from build123d import *

# Parameters (mm, degrees)
SKETCH1_R           = 12.5
BOSS_EXTRUDE1_DEPTH = 3
SKETCH3_R           = 5
BOSS_EXTRUDE2_DEPTH = 3
CUT_EXTRUDE1_DEPTH  = 10


with BuildPart() as part:
    # Sketch1 → Boss-Extrude1 (new body)
    with BuildSketch(Plane(origin=(0, 0, 0), x_dir=(1, 0, 0), z_dir=(0, 1, 0))):
        Circle(SKETCH1_R)
    extrude(amount=BOSS_EXTRUDE1_DEPTH)

    # Sketch3 → Boss-Extrude2 (add)
    with BuildSketch(Plane(origin=(0, 3, 0), x_dir=(1, 0, 0), z_dir=(0, 1, 0))):
        with Locations((0, 11)):
            Circle(SKETCH3_R)
    extrude(amount=-BOSS_EXTRUDE2_DEPTH)

    # Sketch4 → Cut-Extrude1 (cut)
    with BuildSketch(Plane(origin=(0, 3, 0), x_dir=(1, 0, 0), z_dir=(0, 1, 0))):
        with BuildLine():
            ThreePointArc((0.6, 6), (0.424264069, 6.424264069), (0, 6.6))
            Line((0, 6.6), (0, 5.4))
            ThreePointArc((0, 5.4), (0.424264069, 5.575735931), (0.6, 6))
        make_face()
        with BuildLine():
            Line((0, 5.4), (0, 6.6))
            ThreePointArc((0, 6.6), (-0.6, 6), (0, 5.4))
        make_face()
        with BuildLine():
            ThreePointArc((0.6, 7.5), (0.424264069, 7.924264069), (0, 8.1))
            Line((0, 8.1), (0, 6.9))
            ThreePointArc((0, 6.9), (0.424264069, 7.075735931), (0.6, 7.5))
        make_face()
        with BuildLine():
            Line((0, 6.9), (0, 8.1))
            ThreePointArc((0, 8.1), (-0.6, 7.5), (0, 6.9))
        make_face()
        with BuildLine():
            ThreePointArc((0.6, 9), (0.424264069, 9.424264069), (0, 9.6))
            Line((0, 9.6), (0, 8.4))
            ThreePointArc((0, 8.4), (0.424264069, 8.575735931), (0.6, 9))
        make_face()
        with BuildLine():
            Line((0, 8.4), (0, 9.6))
            ThreePointArc((0, 9.6), (-0.6, 9), (0, 8.4))
        make_face()
        with BuildLine():
            ThreePointArc((0.6, 10.5), (0.424264069, 10.924264069), (0, 11.1))
            Line((0, 11.1), (0, 9.9))
            ThreePointArc((0, 9.9), (0.424264069, 10.075735931), (0.6, 10.5))
        make_face()
        with BuildLine():
            Line((0, 9.9), (0, 11.1))
            ThreePointArc((0, 11.1), (-0.6, 10.5), (0, 9.9))
        make_face()
        with BuildLine():
            ThreePointArc((0.6, 12), (0.424264069, 12.424264069), (0, 12.6))
            Line((0, 12.6), (0, 11.4))
            ThreePointArc((0, 11.4), (0.424264069, 11.575735931), (0.6, 12))
        make_face()
        with BuildLine():
            Line((0, 11.4), (0, 12.6))
            ThreePointArc((0, 12.6), (-0.6, 12), (0, 11.4))
        make_face()
        with BuildLine():
            ThreePointArc((0.6, 13.5), (0.424264069, 13.924264069), (0, 14.1))
            Line((0, 14.1), (0, 12.9))
            ThreePointArc((0, 12.9), (0.424264069, 13.075735931), (0.6, 13.5))
        make_face()
        with BuildLine():
            Line((0, 12.9), (0, 14.1))
            ThreePointArc((0, 14.1), (-0.6, 13.5), (0, 12.9))
        make_face()
        with BuildLine():
            ThreePointArc((0.6, 15), (0.424264069, 15.424264069), (0, 15.6))
            Line((0, 15.6), (0, 14.4))
            ThreePointArc((0, 14.4), (0.424264069, 14.575735931), (0.6, 15))
        make_face()
        with BuildLine():
            Line((0, 14.4), (0, 15.6))
            ThreePointArc((0, 15.6), (-0.6, 15), (0, 14.4))
        make_face()
    extrude(amount=-CUT_EXTRUDE1_DEPTH, mode=Mode.SUBTRACT)


solid = part.part
Geometry: final body of the model. Coordinates: model frame, mm. Round coordinates to 2 decimals unless told otherwise and drop trailing zeros. Order: outer loops, then holes, each group sorted by start corner. A loop starts at its lowest first (then second) coordinate and runs counter-clockwise, first axis right, second up. Notation, with made-up numbers: (-40, -26) - (-25, -26) arc R11 ccw to (-25, -9) - close; hole circle Ø1 at (-9.5, -18). An arc over 180 degrees is marked (long way). Write each question's results on one line, items separated by ' | '.
Item 1: First-contact query: pin 1 Ø1 at (y, z) = (2.5, -10) entering from -X. Flat tip, straight axial feed; report the tip coordinate or a pass-through.
Completed:
pin 1: x = -8.12
Item 2: Section A-A, the plane y = 0.4. Return the cut outline in (x, z).
Completed:
outline: (-4.98, -11.47) arc R5 ccw to (4.98, -11.47) arc R12.5 ccw (long way) to start; hole circle Ø1.2 at (0, -15); hole circle Ø1.2 at (0, -13.5); hole circle Ø1.2 at (0, -12); hole circle Ø1.2 at (0, -10.5); hole circle Ø1.2 at (0, -9); hole circle Ø1.2 at (0, -7.5); hole circle Ø1.2 at (0, -6)
Item 3: Section B-B, the plane z = 5.5. Return the cut outline in (x, y).
Completed:
outline: (-11.22, 0) - (11.22, 0) - (11.22, 3) - (-11.22, 3) - close
Item 4: Section C-C, the plane x = -7. Return the cut outline in (y, z), and give its area (3 significant figures).
Completed:
outline: (0, -10.36) - (3, -10.36) - (3, 10.36) - (0, 10.36) - close | area: 62.1 mm^2
Item 5: Material intervals for line 1 along X through (y, z) = (2.1, -13.75); line 2 along X through (y, z) = (1.7, -11); line 3 along X through (y, z) = (0.7, -11.25), sorted ascending. Write a range as [from, to].
Completed:
line 1: [-4.18, -0.55], [0.55, 4.18] | line 2: [-5.94, -0.33], [0.33, 5.94] | line 3: [-5.45, 5.45]
